Input: part model. Units: mm. Frame: model coordinates. Face numbers are marked on the shaded views. A direction names the side the tool comes from. Give positions to 0.01 mm unless a question says otherwise; leave off trailing zeros. Order: outer loops, then holes, each group sorted by start corner. A loop starts at its lowest first (then second) coordinate and runs counter-clockwise, first axis right, second up. Notation, with made-up numbers: M 43.25,22.25 L 57.25,22.25 A19 ccw 57.25,39.25 Z; hole C -21,-22.75 d9. An arc over 180 degrees is marked long. Use a Markdown table: item, result.
from build123d import *


with BuildPart() as f2:
    # F2: sweep along a path in F0
    with BuildLine(Plane.XZ) as f2_path:
        Line((0, 0), (0, 34.8548106849))
        Line((0, 34.8548106849), (-5.8264764957, 41.9298186898))
        Line((-5.8264764957, 41.9298186898), (-16.6470743716, 41.9298186898))
        Line((-16.6470743716, 41.9298186898), (-22.4735494703, 34.8548106849))
        Line((-22.4735494703, 34.8548106849), (-22.4735494703, 29.2364228517))
    # F1 (on Top) → F2 (sweep)
    with BuildSketch(Plane.XY):
        Polygon((-4.2523382608, -13.0273997208), (13.4082282339, 2.831066901), (-9.155889973, 10.1963328198), align=None)
    sweep(path=f2_path.line, transition=Transition.RIGHT)


solid = f2.part
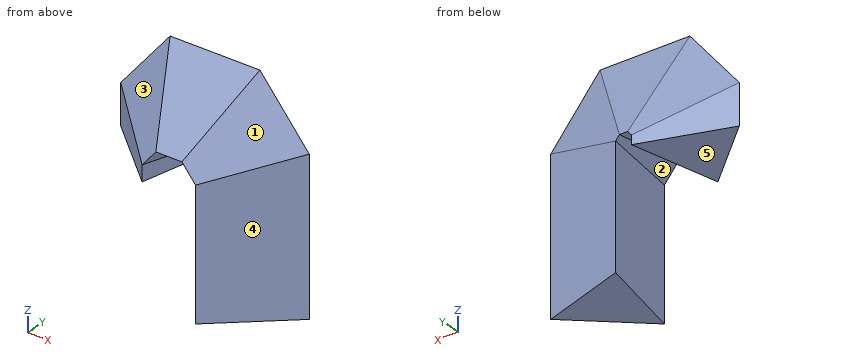
1) Material intervals for line 1 (X direction, y = -10.5, z = 35); line 2 (Z direction, x = -1.5, y = -10.5); line 3 (X direction, y = -4, z = 13), sorted ascending. Write a range as from..to.
Response values:
| item | result |
|---|---|
| line 1 | x = -20.49..-16.15, -6.32..-1.98 |
| line 2 | z = 0..34.41 |
| line 3 | x = -6.16..5.8 |
2) First-contact query: pin 1 Ø11.5 at (x, y) = (-27.5, 3.5) entering from -Z; pin 2 Ø3 at (y, z) = (1.5, 36.5) entering from +X; pin 3 Ø3 at (y, z) = (4, 32.5) entering from -X. Flat tips, straight axial feed; report the tip coordinate or a pass-through.
Response values:
| item | result |
|---|---|
| pin 1 | stops at z = 29.24 |
| pin 2 | stops at x = 13.41 |
| pin 3 | stops at x = -35.88 |
3) Cut plane D-D on x = -31. Return loops of the section in (y, z).
Response values:
| item | result |
|---|---|
| outline | M -1.55,29.24 L 4.42,29.24 L 4.42,37.91 L 2.83,45.59 L -1.55,37.91 Z |
4) Cut plane B-B on z = 35.5. Return loops of the section in (x, y).
Response values:
| item | result |
|---|---|
| outline | M -35.88,2.83 L -24.27,-7.59 L -16.43,-13.03 L -13.61,-2.71 L -8.86,-2.71 L -6.04,-13.03 L 1.8,-7.59 L 13.41,2.83 L 1.8,6.62 L -8.86,9.31 L -13.61,9.31 L -24.27,6.62 Z |
5) Reachability of the marked faces 4 and 5 from +Z, -Z, +X, -X, +Y, -Y: full face, straight path, thin tool, end or side. Return the list, or none.
Response values:
| item | result |
|---|---|
| face 4 | +Z, -Z, +X, -Y |
| face 5 | -Z, -X, +Y, -Y |
6) Cut plane C-C on x = -17. Return loops of the section in (y, z).
Response values:
| item | result |
|---|---|
| outline | M -13.03,34.81 L -7.24,32.89 L -7.24,29.24 L 8.99,29.24 L 8.99,32.89 L 6.96,42.68 L 2.83,55.34 L -8.54,42.68 Z |
7) Cut plane A-A on y = -9.75. Return loops of the section in (x, z).
Response values:
| item | result |
|---|---|
| outline | M -21.87,29.24 L -17.53,29.24 L -17.53,33.08 L -14.31,36.99 L -8.16,36.99 L -4.94,33.08 L -4.94,0 L -0.6,0 L -0.6,34.64 L -6.11,41.33 L -16.36,41.33 L -21.87,34.64 Z |
8) Mould query, pull axis X, two halves, no side actions, for the marked faces 1, 2 and 3. Classes: released by +X, released by -X, zero draft, split by the parting line, or undercut.
Response values:
| item | result |
|---|---|
| face 1 | released by +X |
| face 2 | undercut |
| face 3 | released by -X |
